Autodesk Inventor part; units mm, degrees
ref_plane "YZ Plane" through (0, 0, 0) normal (1, 0, 0) x (0, 1, 0)
ref_plane "XZ Plane" through (0, 0, 0) normal (0, 1, 0) x (-1, 0, 0)
ref_plane "XY Plane" through (0, 0, 0) normal (0, 0, 1) x (1, 0, 0)
sketch "Sketch1" plane through (0, 0, 0) normal (0, 1, 0) x (-1, 0, 0)
  line L0 (0, 0) -> (14, 0)
  line L1 (14, 0) -> (14, -2)
  line L2 (14, -2) -> (0, -2)
  line L3 (0, -2) -> (0, 0)
  line L4 (14, -1) -> (13, -1)
  line L5 (7, -2) -> (7, -1)
  circle A0 centre (13, -1) radius 0.5
  circle A1 centre (1, -1) radius 0.5
  dimension "d0" = 14
  dimension "d1" = 2
  dimension "d2" = 1
  dimension "d3" = 1
extrude "Extrusion1" add sketch "Sketch1" along normal blind 8
sketch "Sketch2" plane through (0, 8, 0) normal (0, 1, 0) x (1, 0, 0)
  circle A0 centre (-13, 1) radius 0.5
  line L0 (-13, 1) -> (-11.5, 1)
  line L1 (-11.5, 1) -> (-11.5, 2)
  line L2 (0, 2) -> (-14, 2)
  line L3 (-11.5, 1) -> (-11.5, 0)
  line L4 (-14, 0) -> (0, 0)
  line L5 (-7, 2) -> (-7, 5.1392)
  line L6 (-13, 1) -> (-11.5, 2)
  line L7 (-13, 1) -> (-11.5, 0)
  circle A1 centre (-1, 1) radius 0.5
  line L8 (-1, 1) -> (-2.5, 1)
  line L9 (-2.5, 1) -> (-2.5, 2)
  line L10 (-14, 2) -> (0, 2)
  line L11 (-2.5, 1) -> (-2.5, 0)
  line L12 (0, 0) -> (-14, 0)
  line L13 (-1, 1) -> (-2.5, 2)
  line L14 (-1, 1) -> (-2.5, 0)
  line L15 (-11.5, 0) -> (-14, 0)
  line L16 (-14, 0) -> (-14, 2)
  line L17 (-14, 2) -> (-11.5, 2)
  line L18 (-11.5, 2) -> (-11.5, 0)
  line L19 (0, 0) -> (0, 2)
  line L20 (0, 0) -> (-2.5, 0)
  line L21 (-2.5, 0) -> (-2.5, 2)
  line L22 (-2.5, 2) -> (0, 2)
  line L23 (0, 2) -> (0, 0)
  point P0 (-12.584, 0.7226)
  point P1 (-12.584, 1.2774)
  point P2 (-1.416, 1.2774)
  point P3 (-1.416, 0.7226)
  dimension "d6" = 1.5
extrude "Extrusion2" add sketch "Sketch2" against normal blind 8 contours L0 L6 A0 | L0 L3 L7 A0 | A0 L7 L0 | A0 L6 L1 L0 | L11 L8 A1 L14 | L13 A1 L8 L9 | A1 L8 L14 | L13 L8 A1
extrude "Extrusion3" cut sketch "Sketch2" against normal blind 8 contours A0 L7 L4 L16 L2 L6 | L14 A1 L13 L2 L19 L4
sketch "Sketch3" plane through (0, 8, 0) normal (0, 1, 0) x (1, 0, 0)
  line L0 (-11.5, 2) -> (-13, 1)
  line L1 (-1, 1) -> (-2.5, 2)
  line L2 (-13, 1) -> (-1, 1)
  line L3 (-13, 1) -> (-11.5, 0)
  line L4 (-13, 1) -> (-0.4084, 1)
  line L5 (-0.4084, 1) -> (-0.4084, 3.5124)
  line L6 (-0.4084, 3.5124) -> (-13, 3.5124)
  line L7 (-13, 3.5124) -> (-13, 1)
  point P0 (0, 0)
extrude "Extrusion4" cut sketch "Sketch3" against normal blind 8
sketch "Sketch4" plane through (0, 8, 0) normal (0, 1, 0) x (1, 0, 0)
  line L0 (-11.5, 0) -> (-11.5, -1)
  line L1 (-11.5, 0) -> (-13, 1)
  line L2 (-11.5, -1) -> (-13, 1)
  line L3 (-11.5, 0) -> (-2.5, 0)
  line L4 (-13, 1) -> (-11.5, 0)
  line L5 (-1, 1) -> (-13, 1)
  line L6 (-7, 1) -> (-7, 2.0592)
  line L7 (-2.5, 0) -> (-2.5, -1)
  line L8 (-2.5, 0) -> (-1, 1)
  line L9 (-2.5, -1) -> (-1, 1)
  line L10 (-1, 1) -> (-2.5, 0)
  line L11 (-11.5, -1) -> (-2.5, -1)
  line L12 (-11.5, 0) -> (-2.5, 0)
  point P0 (0, 0)
  dimension "d13" = 1
extrude "Extrusion5" add sketch "Sketch4" against normal blind 8 contours L3 L7 L11 L0 | L0 L2 L1 | L8 L9 L7
properties part number "link_v2"
Could you check a few things on this model? Use its own coordinates, in mm. Give positions to 0.01 mm unless a question says otherwise; leave off trailing zeros. Loops run counter-clockwise (first coordinate to the right, second up) from the corner with the lowest first, then second, coordinate; pieces in that order, holes last. Notation, with made-up numbers: M 40,18 L 54,18 A22 ccw 54,56 Z; hole C 62.25,-21.5 d5. An arc over 180 degrees is marked long. Answer as a JSON object with one key per item and string values.
Q1. Suppose I cut it at B-B, the plane y = 2. List the corners of the cut face in (x, z) for me.
Values found:
{"outline": "M -13,-1 L -1,-1 L -2.5,1 L -11.5,1 Z"}
Q2. Suppose I cut it at A-A, the plane z = 0.8. List the corners of the cut face in (x, y) for me.
Values found:
{"outline": "M -11.65,0 L -2.35,0 L -2.35,8 L -11.65,8 Z"}
Q3. For P1, Ø1, axis at y = 5.5, z = 0.5, coming from the +X side, with a flat end and sliding along its axis, tell me the tip position at first contact or that it passes through.
Values found:
{"P1": "stops at x = -1.75"}
Q4. If I drill on probe 1 along X at (y, z) = (0.75, 0.45); probe 2 along X at (y, z) = (3.5, -0.5) (3 decimals); probe 3 along Z at (x, y) = (-12, 4), over which ranges is the centre line in solid material (lowest first)? Write a range as [from, to].
Values found:
{"probe 1": "x = [-11.91, -2.09]", "probe 2": "x = [-12.625, -1.375]", "probe 3": "z = [-1, 0.33]"}
